```python
from build123d import *

# Parameters (mm, degrees)
F1_R            = 3
F1_R_2          = 1.5
F2_DEPTH        = 6
F3_R            = 5
F4_R            = 3
F5_DEPTH        = 12.5
F5_COPIES_COUNT = 3


# Not quite as in the source:
# - a pattern or mirror of a feature is missing from the dataset's text; its kind, count and spacing are read off the source's solid


with BuildPart() as f2:
    # F1 (on Top) → F2 (new body)
    with BuildSketch(Plane.XY):
        with BuildLine():
            ThreePointArc((4.3301270189, 102.5), (4.8296291314, 101.2940952255), (5, 100))
            ThreePointArc((5, 100), (-1.2940952255, 95.1703708686), (-4.3301270189, 102.5))
            Line((-4.3301270189, 102.5), (-90.9326673974, -47.5))
            ThreePointArc((-90.9326673974, -47.5), (-85.3084451529, -45.1703708686), (-81.6025403784, -50))
            ThreePointArc((-81.6025403784, -50), (-83.0670064725, -53.5355339059), (-86.6025403784, -55))
            Line((-86.6025403784, -55), (86.6025403784, -55))
            ThreePointArc((86.6025403784, -55), (82.2724133595, -47.5), (90.9326673974, -47.5))
            Line((90.9326673974, -47.5), (4.3301270189, 102.5))
        make_face()
        with Locations((-38.9711431703, 22.5)):
            Circle(F1_R, mode=Mode.SUBTRACT)
        with Locations((0, -45)):
            Circle(F1_R, mode=Mode.SUBTRACT)
        Polygon((60.6217782649, -35), (-60.6217782649, -35), (0, 70), align=None, mode=Mode.SUBTRACT)
        with Locations((38.9711431703, 22.5)):
            Circle(F1_R, mode=Mode.SUBTRACT)
        with BuildLine():
            ThreePointArc((91.6025403784, -50), (91.4321695099, -48.7059047745), (90.9326673974, -47.5))
            ThreePointArc((90.9326673974, -47.5), (82.2724133595, -47.5), (86.6025403784, -55))
            ThreePointArc((86.6025403784, -55), (90.1380742844, -53.5355339059), (91.6025403784, -50))
        make_face()
        with Locations((86.6025403784, -50)):
            Circle(F1_R_2, mode=Mode.SUBTRACT)
        with BuildLine():
            ThreePointArc((-81.6025403784, -50), (-85.3084451529, -45.1703708686), (-90.9326673974, -47.5))
            ThreePointArc((-90.9326673974, -47.5), (-90.9326673974, -52.5), (-86.6025403784, -55))
            ThreePointArc((-86.6025403784, -55), (-83.0670064725, -53.5355339059), (-81.6025403784, -50))
        make_face()
        with Locations((-86.6025403784, -50)):
            Circle(F1_R_2, mode=Mode.SUBTRACT)
        with BuildLine():
            ThreePointArc((-4.3301270189, 102.5), (-1.2940952255, 95.1703708686), (5, 100))
            ThreePointArc((5, 100), (4.8296291314, 101.2940952255), (4.3301270189, 102.5))
            ThreePointArc((4.3301270189, 102.5), (0, 105), (-4.3301270189, 102.5))
        make_face()
        with Locations((0, 100)):
            Circle(F1_R_2, mode=Mode.SUBTRACT)
    extrude(amount=F2_DEPTH)

    # F3
    f3_edges = [f2.edges().sort_by_distance(p)[0] for p in [
        (0, 70, 3),
        (-60.621778, -35, 3),
        (60.621778, -35, 3),
    ]]
    fillet(f3_edges, radius=F3_R)

    # F4 (on Top) → F5 (cut, symmetric)
    with BuildSketch(Plane.XY):
        with Locations((0, 87.5)):
            Circle(F4_R)
    f5 = extrude(amount=F5_DEPTH, both=True, mode=Mode.SUBTRACT)

    # F5_copies: F5 ×3 about axis
    f5_copies_axis = Axis((0, 0, 0), (0, 0, 1))
    for i in range(1, F5_COPIES_COUNT):
        add(f5.rotate(f5_copies_axis, i * 360 / F5_COPIES_COUNT), mode=Mode.SUBTRACT)


solid = f2.part
```
The model under review builds one solid part; all positions refer to its coordinate system, in mm. A direction names the side the tool comes from. Round coordinates to 2 decimals unless told otherwise and drop trailing zeros. Loops run counter-clockwise (first coordinate to the right, second up) from the corner with the lowest first, then second, coordinate; pieces in that order, holes last. Notation, with made-up numbers: (13.25, 6.5) - (61.25, 6.5) arc R20 ccw to (61.25, 44.5) - close; hole circle Ø4 at (38.5, 18.25). An arc over 180 degrees is marked (long way). Write each question's results on one line, items separated by ' | '. Start each with the question number.
Q1. Take a section at A-A on x = -50. Give the boundary of the cut face in (y, z), plus the area to 3 significant figures.
Q2. Draft analysis for pull direction X (two halves, no side actions). For faces 3 (the cylindrical face through (-56.328, -32.436, 3.042)), 4 (the flat face through (-34, 19, 0)), 5 (the flat face through (-30.675, 16.87, 2.958)), 6 (the cylindrical face through (0, 105, 3)), state which applies: pulls with the +X half, pulls with the -X half, needs draft (parallel to the pull), parting line crosses it, or undercut.
Q3. Take a section at C-C on y = 87.5. Give the boundary of the cut face in (x, z).
Q4. Take a section at B-B on y = 22.5. Give the boundary of the cut face in (x, z).
Q5. Insertion check: P1, Ø3, axis at x = -5, z = 2.5, coming from the +Y side; P2, Ø1.5, axis at y = 9.5, z = 3, coming from the +X side. Each pin has a flat end and moves straight along its axis. Give the tip position at first contact, or say it passes through.
Q6. Tool access review of faces 1 (the flat face through (-47.025, 28.55, 2.958)), 2 (the cylindrical face through (0, 65, 3)): name each direction out of +Z, -Z, +X, -X, +Y, -Y from which nothing blocks a thin tool from reaching the whole face with its end or side.
Q7. Wall thickness on line 1 along Y through (x, z) = (-39, 4); line 2 along Y through (x, z) = (36.5, 4.9); line 3 along X through (y, z) = (39, 1.3): over which ranges is each line inside the solid? List them lowest first. Write a range as [from, to].
Q8. Take a section at D-D on z = 1.9. Give the number of separate pieces and of enclosed holes in the cut face, plus the area to 3 significant figures.
Data:
1) outline: (-55, 0) - (-35, 0) - (-35, 6) - (-55, 6) - close; (-16.6, 0) - (23.4, 0) - (23.4, 6) - (-16.6, 6) - close | area: 360 mm²
2) face 3: undercut | face 4: needs draft | face 5: undercut | face 6: parting line crosses it
3) outline: (-12.99, 0) - (-3, 0) - (-3, 6) - (-12.99, 6) - close; (3, 0) - (12.99, 0) - (12.99, 6) - (3, 6) - close
4) outline: (-50.52, 0) - (-41.97, 0) - (-41.97, 6) - (-50.52, 6) - close; (-35.97, 0) - (-27.42, 0) - (-27.42, 6) - (-35.97, 6) - close; (27.42, 0) - (35.97, 0) - (35.97, 6) - (27.42, 6) - close; (41.97, 0) - (50.52, 0) - (50.52, 6) - (41.97, 6) - close
5) P1: stops at y = 103.57 | P2: stops at x = 58.46
6) face 1: +Z, -Z, -X, +Y | face 2: +Z, -Z
7) line 1: y = [-55, -35], [2.45, 19.5], [25.5, 42.45] | line 2: y = [-55, -35], [6.78, 20.8], [24.2, 46.78] | line 3: x = [-40.99, -17.9], [17.9, 40.99]
8) separate pieces: 1 | enclosed holes: 10 | area: 9,160 mm²
